from build123d import *

# Parameters (mm, degrees)
F0_R     = 10
F1_DEPTH = 7
F2_R     = 3
F3_DEPTH = 9
F4_R     = 3
F5_R     = 0.5


with BuildPart() as f1:
    # F0 (on Top) → F1 (new body)
    with BuildSketch(Plane.XY):
        Circle(F0_R)
    extrude(amount=-F1_DEPTH)

    # F2 (on face) → F3 (join)
    with BuildSketch(Plane.XY):
        Circle(F2_R)
    extrude(amount=F3_DEPTH)

    # F4
    f4_edges = [f1.edges().sort_by_distance(p)[0] for p in [
        (-10, 0, -7),
    ]]
    fillet(f4_edges, radius=F4_R)

    # F5
    f5_edges = [f1.edges().sort_by_distance(p)[0] for p in [
        (-10, 0, 0),
        (-3, 0, 9),
        (-3, 0, 0),
    ]]
    fillet(f5_edges, radius=F5_R)


solid = f1.part
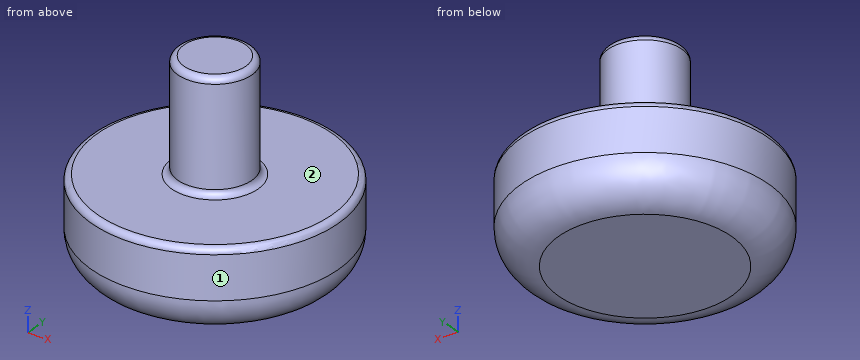
For this review, take the finished solid that the model builds, in its own axes (mm). Face numbers are marked on the shaded views. A direction names the side the tool comes from. Give positions to 0.01 mm unless a question says otherwise; leave off trailing zeros. Write each loop counter-clockwise with the first axis right and the second up, starting at its lowest first coordinate (ties: lowest second). Pieces come first, ordered by that corner, then holes. Notation, with made-up numbers: (34, -35) -> (42, -35) arc R22 cw to (42, -3) -> close; hole circle Ø10 at (42, 29.5). An arc over 180 degrees is marked (long way). Use CSV: the item, a comma, the result in double quotes.
Q1. Take a section at C-C, the plane z = 7. Write out the cut boundary in (x, y).
Conclusion:
outline,"circle Ø6 at (0, 0)"
Q2. For P1, Ø5, axis at x = 5.5, z = 1, coming from the -Y side; P2, Ø1.5, axis at y = 2, z = 7, coming from the -X side; P3, Ø3, axis at y = -3.5, z = 6.5, coming from the -X side, all flat-tipped, find the tip position at first contact; note any pin that passes through.
Conclusion:
P1,"y = -9.38"
P2,"x = -2.73"
P3,"x = -2.24"
Q3. Take a section at A-A, the plane x = 0. Write out the cut boundary in (y, z).
Conclusion:
outline,"(-10, -4) arc R3 ccw to (-7, -7) -> (7, -7) arc R3 ccw to (10, -4) -> (10, -0.5) arc R0.5 ccw to (9.5, 0) -> (3.5, 0) arc R0.5 cw to (3, 0.5) -> (3, 8.5) arc R0.5 ccw to (2.5, 9) -> (-2.5, 9) arc R0.5 ccw to (-3, 8.5) -> (-3, 0.5) arc R0.5 cw to (-3.5, 0) -> (-9.5, 0) arc R0.5 ccw to (-10, -0.5) -> close"
Q4. Tool access review of the marked faces 1 and 2: name each direction out of +Z, -Z, +X, -X, +Y, -Y from which nothing blocks a thin tool from reaching the whole face with its end or side.
Conclusion:
face 1,"+Z, -Z"
face 2,"+Z"
Q5. To check wall thickness, follow probe 1 along Z at (x, y) = (-5, -3); probe 2 along Z at (x, y) = (-7.75, 0.25); probe 3 along X at (y, z) = (3, -5.25). State the ranges of each line that lie inside material, in increasing order. Write a range as [from, to].
Conclusion:
probe 1,"[-7, 0]"
probe 2,"[-6.9, 0]"
probe 3,"[-9.25, 9.25]"
